```python
from build123d import *

# Parameters (mm, degrees)
F0_R             = 67.8801752346
F1_DEPTH         = 12.7
F2_R             = 9.6644171041
F3_DEPTH         = 25.4
F3_COPIES_COUNT  = 16
F4_R             = 7.2675454898
F5_DEPTH         = 31.75
F5_COPIES_COUNT  = 13
F6_R             = 5.0242913047
F7_DEPTH         = 38.1
F7_COPIES_COUNT  = 11
F8_R             = 3.0016652879
F9_DEPTH         = 50.8
F9_COPIES_COUNT  = 9
F10_R            = 1.9805186859
F11_DEPTH        = 101.6
F11_COPIES_COUNT = 5


# Not quite as in the source:
# - a pattern or mirror of a feature is missing from the dataset's text; its kind, count and spacing are read off the source's solid


with BuildPart() as f1:
    # F0 (on Top) → F1 (new body, symmetric)
    with BuildSketch(Plane.XY):
        Circle(F0_R)
    extrude(amount=F1_DEPTH, both=True)

    # F2 (on face) → F3 (join)
    with BuildSketch(Plane.XY.offset(12.7)):
        with Locations((-32.3193110526, 38.2313802838)):
            Circle(F2_R)
    f3 = extrude(amount=F3_DEPTH)

    # F3_copies: F3 ×16 about axis
    f3_copies_axis = Axis((0, 0, 0), (0, 0, 1))
    for i in range(1, F3_COPIES_COUNT):
        add(f3.rotate(f3_copies_axis, i * 360 / F3_COPIES_COUNT))

    # F4 (on face) → F5 (join)
    with BuildSketch(Plane.XY.offset(12.7)):
        with Locations((-19.9039652944, 25.22482723)):
            Circle(F4_R)
    f5 = extrude(amount=F5_DEPTH)

    # F5_copies: F5 ×13 about axis
    f5_copies_axis = Axis((0, 0, 0), (0, 0, 1))
    for i in range(1, F5_COPIES_COUNT):
        add(f5.rotate(f5_copies_axis, i * 360 / F5_COPIES_COUNT))

    # F6 (on face) → F7 (join)
    with BuildSketch(Plane.XY.offset(12.7)):
        with Locations((-11.4300008863, 13.7948282063)):
            Circle(F6_R)
    f7 = extrude(amount=F7_DEPTH)

    # F7_copies: F7 ×11 about axis
    f7_copies_axis = Axis((0, 0, 0), (0, 0, 1))
    for i in range(1, F7_COPIES_COUNT):
        add(f7.rotate(f7_copies_axis, i * 360 / F7_COPIES_COUNT))

    # F8 (on face) → F9 (join)
    with BuildSketch(Plane.XY.offset(12.7)):
        with Locations((-6.1091380194, 7.2915516794)):
            Circle(F8_R)
    f9 = extrude(amount=F9_DEPTH)

    # F9_copies: F9 ×9 about axis
    f9_copies_axis = Axis((0, 0, 0), (0, 0, 1))
    for i in range(1, F9_COPIES_COUNT):
        add(f9.rotate(f9_copies_axis, i * 360 / F9_COPIES_COUNT))

    # F10 (on face) → F11 (join)
    with BuildSketch(Plane.XY.offset(12.7)):
        with Locations((-2.36482732, 2.5618965738)):
            Circle(F10_R)
    f11 = extrude(amount=F11_DEPTH)

    # F11_copies: F11 ×5 about axis
    f11_copies_axis = Axis((0, 0, 0), (0, 0, 1))
    for i in range(1, F11_COPIES_COUNT):
        add(f11.rotate(f11_copies_axis, i * 360 / F11_COPIES_COUNT))


solid = f1.part
```
The listing builds one solid part. Answer for the finished solid, in the listing's coordinates (mm). A direction names the side the tool comes from. Coordinates: 2 decimals unless noted, no trailing zeros. Loops run counter-clockwise (first coordinate to the right, second up) from the corner with the lowest first, then second, coordinate; pieces in that order, holes last. Notation, with made-up numbers: M 55.5,7 L 99.5,7 A18 ccw 99.5,20 Z; hole C 53,85.5 d2. An arc over 180 degrees is marked long. Answer as a JSON object with one key per item and string values. Group by question number.
Item 1: Determine the mould class of faces 1 (the face through (14.39, -38.06, 25.22)), 2 (the face through (48, 15, 38.1)) for opening direction Y: +Y half, -Y half, draft (parallel to the pull), parting line (faces both ways), or undercut.
Item 2: Consider L1, parallel to X at y = -9, z = 57.5; L2, parallel to Y at x = -34, z = 18.5; L3, parallel to Y at x = 50, z = 32.5. Determine where each line is inside the solid, lowest interval first.
Item 3: Which of the six approach directions +Z, -Z, +X, -X, +Y, -Y give full straight-line access (tool end or side, diameter ignored) to faces 3 (the face through (-50, 4, 38.1)), 4 (the face through (3, -9, 63.5)), 5 (the face through (-45, 23, 38.1)), 6 (the face through (-14.39, 38.06, 25.22))?
Item 4: Each of these flat-tipped pins is pushed along its axis until it touches: P1, Ø11.5, axis at x = -25.5, y = 15.5, coming from the +Z side; P2, Ø5, axis at x = -19.5, y = -4, coming from the +Z side; P3, Ø21.5, axis at x = -15, y = 47.5, coming from the +Z side. Where does it stop, or does it pass through?
Item 5: Section A-A (z = 78) is taken. Write down the section's boundary in (x, y).
Item 6: Section C-C (y = 50.5) is taken. Write down the section's boundary in (x, z), and give its area (3 significant figures).
Item 7: Section B-B (z = 55) is taken. Give the number of separate pieces and of enclosed holes in the cut face, and give its area (3 significant figures).
Solved:
{
 "1": {"face 1": "undercut", "face 2": "draft"},
 "2": {"L1": "x = -6.26 to -0.26, 0.25 to 6.25", "L2": "y = -41.01 to -23.63, -19.85 to -13.59, -9.06 to 4.95, 7.5 to 18.67, 28.71 to 47.75", "L3": "y = -30.89 to -15.01, -13.84 to 5.48, 5.84 to 24.61"},
 "3": {"face 3": "+Z, -X, +Y, -Y", "face 4": "+Z, +X, -X, -Y", "face 5": "+Z, -X, +Y", "face 6": "+Z"},
 "4": {"P1": "stops at z = 44.45", "P2": "stops at z = 50.8", "P3": "stops at z = 38.1"},
 "5": {"outline": "C -3.17,-1.46 d3.96; C -2.36,2.56 d3.96; C 0.41,-3.46 d3.96; C 1.71,3.04 d3.96; C 3.42,-0.68 d3.96"},
 "6": {"outline": "M -45.36,-12.7 L 45.36,-12.7 L 45.36,12.7 L 30.52,12.7 L 30.52,38.1 L 15.38,38.1 L 15.38,12.7 L 13.83,12.7 L 13.83,38.1 L -5.46,38.1 L -5.46,12.7 L -5.98,12.7 L -5.98,38.1 L -24.48,38.1 L -24.48,12.7 L -45.36,12.7 Z", "area": "3,650 mm2"},
 "7": {"separate pieces": "14", "enclosed holes": "0", "area": "316 mm2"}
}
